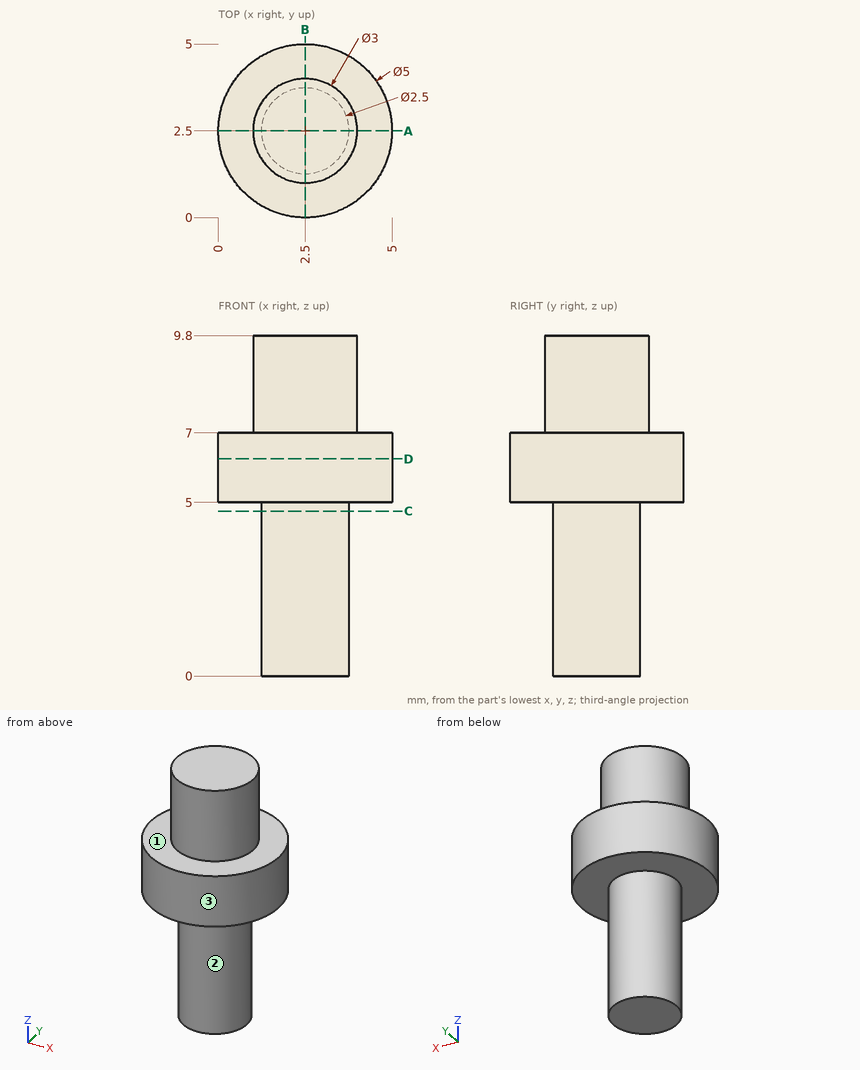
Source: three-view drawing plus pictorial views. Frame: mm from the lowest corner of the part. A direction names the side the tool comes from. Round coordinates to 2 decimals unless told otherwise and drop trailing zeros. Loops run counter-clockwise (first coordinate to the right, second up) from the corner with the lowest first, then second, coordinate; pieces in that order, holes last. Notation, with made-up numbers: M 19,34.5 L 38,34.5 A14 cw 38,47.5 Z; hole C -5,64.25 d6. An arc over 180 degrees is marked long. Put each result on its own line as item: value.
(1) Access query for the marked faces 1, 2 and 3. Directions: +Z, -Z, +X, -X, +Y, -Y. A direction counts if a zero-diameter tool reaches every point of the face in a straight line with its end or side. Return the directions, or none.
Solutions:
face 1: +Z
face 2: -Z
face 3: +Z, -Z
(2) First-contact query: pin 1 (1 mm diameter, centred on x = 4, y = 3, fed in from -Z); pin 2 (1.5 mm diameter, centred on x = 4, z = 2.5, fed in from -Y); pin 3 (3 mm diameter, centred on x = 2, z = 2.5, fed in from +Y); pin 4 (1 mm diameter, centred on x = 1.5, z = 2, fed in from -Y). Flat tips, straight axial feed; report the tip coordinate or a pass-through.
Solutions:
pin 1: z = 0
pin 2: y = 1.5
pin 3: y = 3.75
pin 4: y = 1.35
(3) Ray query, line 1 (Z direction, x = 1.35, y = 4.5); line 2 (Y direction, x = 2.15, z = 6); line 3 (Z direction, x = 2.65, y = 3.8). Return the intervals inside material, ascending. Write a range as [from, to].
Solutions:
line 1: [5, 7]
line 2: [0.02, 4.98]
line 3: [5, 9.8]
(4) Section D-D, the plane z = 6.25. Return loops of the section in (x, y), and give its area (3 significant figures).
Solutions:
outline: C 2.5,2.5 d5
area: 19.6 mm²
(5) Section A-A, the plane y = 2.5. Return loops of the section in (x, z).
Solutions:
outline: M 0,5 L 1.25,5 L 1.25,0 L 3.75,0 L 3.75,5 L 5,5 L 5,7 L 4,7 L 4,9.8 L 1,9.8 L 1,7 L 0,7 Z
(6) Section C-C, the plane z = 4.75. Return loops of the section in (x, y), and give its area (3 significant figures).
Solutions:
outline: C 2.5,2.5 d2.5
area: 4.91 mm²
